Geometry: see drawing. Coordinates: mm, zero at the bounding-box minimum. A direction names the side the tool comes from. Give positions to 0.01 mm unless a question says otherwise; leave off trailing zeros. Order: outer loops, then holes, each group sorted by start corner. A loop starts at its lowest first (then second) coordinate and runs counter-clockwise, first axis right, second up. Notation, with made-up numbers: (40.25, -4) - (62.25, -4) arc R16 ccw to (62.25, 6) - close; hole circle Ø9 at (46.25, 68). An arc over 180 degrees is marked (long way). One line per item, written item: value. Start each with the question number.
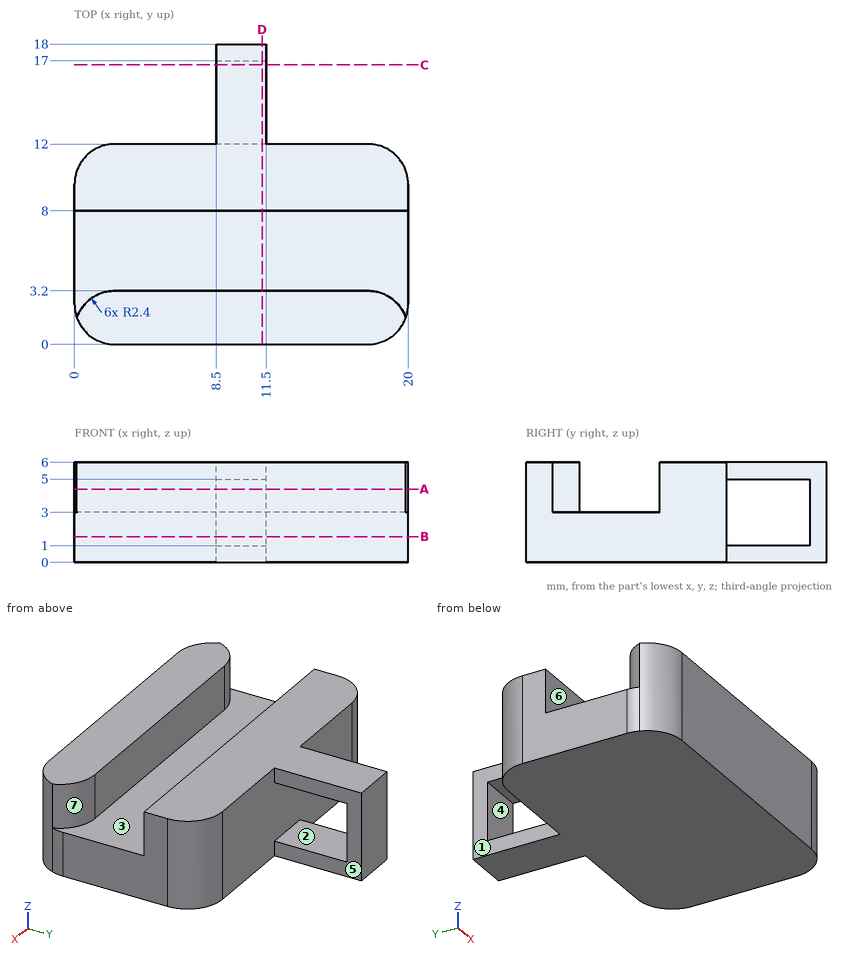
1. Section C-C on y = 16.75. Return the cut outline in (x, z).
2. Set-up query: the marked faces 4, 5, 6 and 7. Return all of +Z, -Z, +X, -X, +Y, -Y with unobstructed straight access to the full face (end or side cutting, diameter ignored); none if empty.
3. Ray query, L1, parallel to Y at x = 10.5, z = 1.55; L2, parallel to Y at x = 16, z = 4.8; L3, parallel to Z at x = 10.25, y = 6.5. Return the intervals inside material, ascending.
4. Contact query for a flat-ended pin moving along its axis: pin 1 Ø2 at (x, z) = (6, 3.5) entering from +Y. Output: stop coordinate, or through.
5. Section A-A on z = 4.4. Return the cut outline in (x, y).
6. Section B-B on z = 1.55. Return the cut outline in (x, y), then the cut area to 3 significant figures.
7. Draft query along Z for the marked faces 1, 2 and 3. Return one class per face: pulls with the +Z half, pulls with the -Z half, needs draft (parallel to the pull), parting line crosses it, or undercut.
8. Section D-D on x = 11.25. Return the cut outline in (y, z).
Data:
1. outline: (8.5, 0) - (11.5, 0) - (11.5, 1) - (8.5, 1) - close; (8.5, 5) - (11.5, 5) - (11.5, 6) - (8.5, 6) - close
2. face 4: +X, -X
2. face 5: +Z, -Z, +X, +Y
2. face 6: +Z, +X, -X
2. face 7: +Z, +X
3. L1: y = 0 to 12, 17 to 18
3. L2: y = 0 to 3.2, 8 to 12
3. L3: z = 0 to 3
4. pin 1: stops at y = 12
5. outline: (0, 8) - (20, 8) - (20, 9.6) arc R2.4 ccw to (17.6, 12) - (2.4, 12) arc R2.4 ccw to (0, 9.6) - close; (0.14, 1.6) arc R2.4 ccw to (2.4, 0) - (17.6, 0) arc R2.4 ccw to (19.86, 1.6) arc R2.4 ccw to (17.6, 3.2) - (2.4, 3.2) arc R2.4 ccw to start; (8.5, 17) - (11.5, 17) - (11.5, 18) - (8.5, 18) - close
6. outline: (0, 2.4) arc R2.4 ccw to (2.4, 0) - (17.6, 0) arc R2.4 ccw to (20, 2.4) - (20, 9.6) arc R2.4 ccw to (17.6, 12) - (2.4, 12) arc R2.4 ccw to (0, 9.6) - close; (8.5, 17) - (11.5, 17) - (11.5, 18) - (8.5, 18) - close
6. area: 238 mm2
7. face 1: needs draft
7. face 2: undercut
7. face 3: pulls with the +Z half
8. outline: (0, 0) - (18, 0) - (18, 6) - (8, 6) - (8, 3) - (3.2, 3) - (3.2, 6) - (0, 6) - close; hole (12, 1) - (17, 1) - (17, 5) - (12, 5) - close
